The model under review builds one solid part; all positions refer to its coordinate system, in mm. Face numbers are marked on the shaded views. A direction names the side the tool comes from. Coordinates: 2 decimals unless noted, no trailing zeros. Write each loop counter-clockwise with the first axis right and the second up, starting at its lowest first coordinate (ties: lowest second). Pieces come first, ordered by that corner, then holes. Notation, with made-up numbers: (89.5, 29) -> (128.5, 29) arc R16 ccw to (128.5, 39) -> close; hole circle Ø9 at (69.25, 6.25). An arc over 180 degrees is marked (long way). Write each question's results on one line, items separated by ' | '.
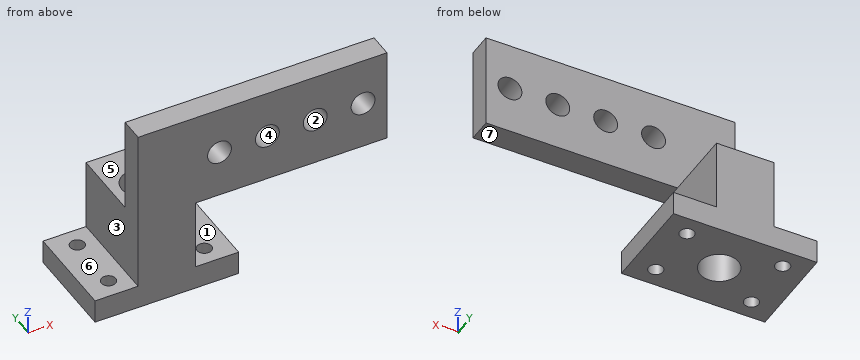
```python
from build123d import *

# Parameters (mm, degrees)
SKETCH_1_W          = 30
SKETCH_1_H          = 20
SKETCH_1_R          = 1.5
SKETCH_1_R_2        = 4
EXTRUDE_1_DEPTH     = 20
SKETCH_2_W          = 9
SKETCH_2_H          = 20
CUT_EXTRUDE_1_DEPTH = 15
SKETCH_3_W          = 12
SKETCH_3_H          = 5
EXTRUDE_2_DEPTH     = 20
SKETCH_4_W          = 20
SKETCH_4_H          = 5
EXTRUDE_3_DEPTH     = 40
SKETCH_5_R          = 2.5
CUT_EXTRUDE_2_DEPTH = 20


with BuildPart() as part:
    # 草图1 → 凸台-拉伸1 (new body)
    with BuildSketch(Plane.XY):
        with Locations((15, -10)):
            Rectangle(SKETCH_1_W, SKETCH_1_H)
        with Locations((5, -4)):
            Circle(SKETCH_1_R, mode=Mode.SUBTRACT)
        with Locations((25, -4)):
            Circle(SKETCH_1_R, mode=Mode.SUBTRACT)
        with Locations((25, -16)):
            Circle(SKETCH_1_R, mode=Mode.SUBTRACT)
        with Locations((5, -16)):
            Circle(SKETCH_1_R, mode=Mode.SUBTRACT)
        with Locations((15, -10)):
            Circle(SKETCH_1_R_2, mode=Mode.SUBTRACT)
    extrude(amount=EXTRUDE_1_DEPTH)

    # 草图2 → 切除-拉伸1 (cut)
    with BuildSketch(Plane.XY.offset(20)):
        with Locations((4.5, -10)):
            Rectangle(SKETCH_2_W, SKETCH_2_H)
        with Locations((25.5, -10)):
            Rectangle(SKETCH_2_W, SKETCH_2_H)
    extrude(amount=-CUT_EXTRUDE_1_DEPTH, mode=Mode.SUBTRACT)

    # 草图3 → 凸台-拉伸2 (add)
    with BuildSketch(Plane.XY.offset(20)):
        with Locations((15, -17.5)):
            Rectangle(SKETCH_3_W, SKETCH_3_H)
    extrude(amount=EXTRUDE_2_DEPTH)

    # 草图4 → 凸台-拉伸3 (add)
    with BuildSketch(Plane(origin=(21, 0, 0), x_dir=(0, 0, -1), z_dir=(1, 0, 0))):
        with Locations((-30, -17.5)):
            Rectangle(SKETCH_4_W, SKETCH_4_H)
    extrude(amount=EXTRUDE_3_DEPTH)

    # 草图5 → 切除-拉伸2 (cut)
    with BuildSketch(Plane(origin=(0, -15, 0), x_dir=(1, 0, 0), z_dir=(0, 1, 0))):
        with Locations((26, -30)):
            Circle(SKETCH_5_R)
        with Locations((36, -30)):
            Circle(SKETCH_5_R)
        with Locations((46, -30)):
            Circle(SKETCH_5_R)
        with Locations((56, -30)):
            Circle(SKETCH_5_R)
    extrude(amount=-CUT_EXTRUDE_2_DEPTH, mode=Mode.SUBTRACT)


solid = part.part
```
Q1. Add section C-C (y = -10). Write out the cut boundary in (x, z).
Solution:
outline: (0, 0) -> (11, 0) -> (11, 20) -> (9, 20) -> (9, 5) -> (0, 5) -> close; (19, 0) -> (30, 0) -> (30, 5) -> (21, 5) -> (21, 20) -> (19, 20) -> close
Q2. Machinability: for the marked faces 5, 6 and 7, which of the approach directions +Z, -Z, +X, -X, +Y, -Y give a long, thin tool a straight path to every point of the face, cutting with its end or side? Answer none if there is none.
Solution:
face 5: +Z, +X, -X, +Y | face 6: +Z, -X, +Y, -Y | face 7: +X, +Y, -Y
Q3. Draft analysis for pull direction X (two halves, no side actions). For the marked faces 1, 2, 3 and 4, state which applies: pulls with the +X half, pulls with the -X half, needs draft (parallel to the pull), parting line crosses it, or undercut.
Solution:
face 1: needs draft | face 2: undercut | face 3: pulls with the -X half | face 4: undercut
Q4. Clearance check with flat-ended pins moving along their axes: P1, Ø10, axis at y = -18, z = 19, coming from the -X side; P2, Ø2, axis at y = -10, z = 19.5, coming from the +X side; P3, Ø5, axis at x = 25, y = -4, coming from the +Z side. State where each tip first meets the part, or that it passes through.
Solution:
P1: x = 9 | P2: x = 21 | P3: z = 5
Q5. For line 1 (X direction, y = -18.3, z = 30); line 2 (Y direction, x = 25, z = 2); line 3 (Z direction, x = 46, y = -17.2), list the stretches that pass through material, from the lowest coordinate up. Write a range as from..to.
Solution:
line 1: 9..23.5, 28.5..33.5, 38.5..43.5, 48.5..53.5, 58.5..61 | line 2: -20..-17.5, -14.5..-5.5, -2.5..0 | line 3: 20..27.5, 32.5..40
Q6. Add section A-A (z = 30). Write out the cut boundary in (x, y).
Solution:
outline: (9, -20) -> (23.5, -20) -> (23.5, -15) -> (9, -15) -> close; (28.5, -20) -> (33.5, -20) -> (33.5, -15) -> (28.5, -15) -> close; (38.5, -20) -> (43.5, -20) -> (43.5, -15) -> (38.5, -15) -> close; (48.5, -20) -> (53.5, -20) -> (53.5, -15) -> (48.5, -15) -> close; (58.5, -20) -> (61, -20) -> (61, -15) -> (58.5, -15) -> close
Q7. Add section B-B (x = 15). Write out the cut boundary in (y, z).
Solution:
outline: (-20, 0) -> (-14, 0) -> (-14, 20) -> (-15, 20) -> (-15, 40) -> (-20, 40) -> close; (-6, 0) -> (0, 0) -> (0, 20) -> (-6, 20) -> close
Q8. Add section D-D (y = -4). Write out the cut boundary in (x, z).
Solution:
outline: (0, 0) -> (3.5, 0) -> (3.5, 5) -> (0, 5) -> close; (6.5, 0) -> (23.5, 0) -> (23.5, 5) -> (21, 5) -> (21, 20) -> (9, 20) -> (9, 5) -> (6.5, 5) -> close; (26.5, 0) -> (30, 0) -> (30, 5) -> (26.5, 5) -> close
